Could you check a few things on this model? Use its own coordinates, in mm. A direction names the side the tool comes from. Round coordinates to 2 decimals unless told otherwise and drop trailing zeros. Loops run counter-clockwise (first coordinate to the right, second up) from the corner with the lowest first, then second, coordinate; pieces in that order, holes last. Notation, with made-up numbers: M 40.5,-9 L 61.5,-9 A34 ccw 61.5,30 Z; hole C 42,39 d9. An arc over 180 degrees is marked long. Return JSON: item names as keys, results as strings. Group by question number.
```python
from build123d import *

# Parameters (mm, degrees)
BODY_EXTRUDE_DEPTH         = 12
M4X0_7_TAPPED_HOLE6_D      = 3.3
CUT_EXTRUDE1_DEPTH         = 32.10064308
M3X0_5_TAPPED_HOLE1_REACH  = 33.101
M3X0_5_TAPPED_HOLE1_BORE_R = 1.25
CHAMFER1_SIZE              = 1


with BuildPart() as part:
    # Body Sketch → Body Extrude (new body)
    with BuildSketch(Plane.XY):
        Polygon((-26.5, 0), (26.5, 0), (26.5, 5), (4.5, 5), (4.5, 11), (-4.5, 11), (-4.5, 5), (-26.5, 5), align=None)
    extrude(amount=-BODY_EXTRUDE_DEPTH)

    # M4x0.7 Tapped Hole6 (through all)
    with Locations(Plane.XZ):
        with Locations((-22.5, -6), (22.5, -6)):
            Hole(M4X0_7_TAPPED_HOLE6_D / 2)

    # Sketch2 → Cut-Extrude1 (cut, through all)
    with BuildSketch(Plane(origin=(0, 0, 0), x_dir=(1, 0, 0), z_dir=(0, 1, 0))):
        with BuildLine():
            Line((-1.581929202, 4), (1.581929202, 4))
            ThreePointArc((1.581929202, 4), (0, 8.55), (-1.581929202, 4))
        make_face()
    extrude(amount=CUT_EXTRUDE1_DEPTH, mode=Mode.SUBTRACT)

    # M3x0.5 Tapped Hole1 bore → M3x0.5 Tapped Hole1 (cut, up to next)
    with BuildSketch(Plane.XY, mode=Mode.PRIVATE) as m3x0_5_tapped_hole1_sk1:
        with Locations((-22.5, 2.5)):
            Circle(M3X0_5_TAPPED_HOLE1_BORE_R)
    m3x0_5_tapped_hole1_tool1 = extrude(m3x0_5_tapped_hole1_sk1.sketch, amount=-M3X0_5_TAPPED_HOLE1_REACH, mode=Mode.PRIVATE) & part.part
    # M3x0.5 Tapped Hole1 bore → M3x0.5 Tapped Hole1 (cut, up to next)
    with BuildSketch(Plane.XY, mode=Mode.PRIVATE) as m3x0_5_tapped_hole1_sk2:
        with Locations((22.5, 2.5)):
            Circle(M3X0_5_TAPPED_HOLE1_BORE_R)
    m3x0_5_tapped_hole1_tool2 = extrude(m3x0_5_tapped_hole1_sk2.sketch, amount=-M3X0_5_TAPPED_HOLE1_REACH, mode=Mode.PRIVATE) & part.part
    # M3x0.5 Tapped Hole1 bore → M3x0.5 Tapped Hole1 (cut, up to next)
    with BuildSketch(Plane.XY, mode=Mode.PRIVATE) as m3x0_5_tapped_hole1_sk3:
        with Locations((0, 8)):
            Circle(M3X0_5_TAPPED_HOLE1_BORE_R)
    m3x0_5_tapped_hole1_tool3 = extrude(m3x0_5_tapped_hole1_sk3.sketch, amount=-M3X0_5_TAPPED_HOLE1_REACH, mode=Mode.PRIVATE) & part.part
    # M3x0.5 Tapped Hole1 bore → M3x0.5 Tapped Hole1 (cut, up to next)
    with BuildSketch(Plane.XY, mode=Mode.PRIVATE) as m3x0_5_tapped_hole1_sk4:
        with Locations((0, 3)):
            Circle(M3X0_5_TAPPED_HOLE1_BORE_R)
    m3x0_5_tapped_hole1_tool4 = extrude(m3x0_5_tapped_hole1_sk4.sketch, amount=-M3X0_5_TAPPED_HOLE1_REACH, mode=Mode.PRIVATE) & part.part
    add(m3x0_5_tapped_hole1_tool1.solids().sort_by_distance((-22.5, 2.5, 0))[0], mode=Mode.SUBTRACT)
    add(m3x0_5_tapped_hole1_tool2.solids().sort_by_distance((22.5, 2.5, 0))[0], mode=Mode.SUBTRACT)
    add(m3x0_5_tapped_hole1_tool3.solids().sort_by_distance((0, 8, 0))[0], mode=Mode.SUBTRACT)
    add(m3x0_5_tapped_hole1_tool4.solids().sort_by_distance((0, 3, 0))[0], mode=Mode.SUBTRACT)

    # Chamfer1
    chamfer1_edges = [part.edges().sort_by_distance(p)[0] for p in [
        (26.5, 2.5, 0),
        (-26.5, 2.5, 0),
        (26.5, 2.5, -12),
        (-26.5, 2.5, -12),
    ]]
    chamfer(chamfer1_edges, length=CHAMFER1_SIZE)


solid = part.part
```
1. If we section it at B-B, the plane x = 22.5: Please give me the cut outline in (y, z).
2. If we section it at A-A, the plane z = -6: Please give me the cut outline in (x, y).
3. I'm going to push flat-ended pins straight in: pin 1 Ø2 at (x, y) = (0, 8) entering from +Z; pin 2 Ø4 at (y, z) = (9.5, -5) entering from +X; pin 3 Ø3 at (y, z) = (7, -5.5) entering from -X. Where does each tip first touch, or does it pass through?
4. We'd pull the mould along Z, two halves only. Please class faces 5 (the face through (0, 11, -3)), 6 (the face through (-22.1, 2.5, -7.6)), 7 (the face through (26, 2.5, -0.5)): +Z half, -Z half, draft (parallel to the pull), parting line (faces both ways), or undercut.
5. I need wall thicknesses on probe 1 along X at (y, z) = (2.75, -3.5); probe 2 along X at (y, z) = (2, -7); probe 3 along Y at (x, z) = (-22.5, -3.5). Which ranges of each line are inside material? Lowest first, please.
6. If we section it at D-D, the plane y = 3: Please give me the cut outline in (x, z), then the cut area to 3 significant figures.
7. If we section it at C-C, the plane x = 0: Please give me the cut outline in (y, z), then the cut area to 4 significant figures.
8. On a 3-axis mill with a long thin cutter (end or side, diameter ignored), from which of +Z, -Z, +X, -X, +Y, -Y can I reach the whole of each face in a straight line? I mean faces 1 (the face through (-0.27, 6.78, -1.97)), 2 (the face through (-15, 5, -6)), 3 (the face through (16, 5, -6)), 4 (the face through (0, 5, -4)). Say none if no direction works.
Geometry results:
{
 "1": {"outline": "M 0,-12 L 5,-12 L 5,-7.65 L 0,-7.65 Z; M 0,-4.35 L 1.25,-4.35 L 1.25,0 L 0,0 Z; M 3.75,-4.35 L 5,-4.35 L 5,0 L 3.75,0 Z"},
 "2": {"outline": "M -26.5,0 L -24.15,0 L -24.15,5 L -26.5,5 Z; M -20.85,0 L -2.55,0 L -2.55,11 L -4.5,11 L -4.5,5 L -20.85,5 Z; M 2.55,0 L 20.85,0 L 20.85,5 L 4.5,5 L 4.5,11 L 2.55,11 Z; M 24.15,0 L 26.5,0 L 26.5,5 L 24.15,5 Z"},
 "3": {"pin 1": "z = -8.35", "pin 2": "x = 4.5", "pin 3": "x = -4.5"},
 "4": {"face 5": "draft", "face 6": "undercut", "face 7": "+Z half"},
 "5": {"probe 1": "-26.5 to -23.72, -21.28 to -1.22, 1.22 to 21.28, 23.72 to 26.5", "probe 2": "-26.5 to -23.81, -21.19 to -2.35, 2.35 to 21.19, 23.81 to 26.5", "probe 3": "0 to 1.25, 3.75 to 5"},
 "6": {"outline": "M -26.5,-11 L -25.5,-12 L 25.5,-12 L 26.5,-11 L 26.5,-1 L 25.5,0 L 23.65,0 L 23.65,-4.81 A1.65 cw long 21.35,-4.81 L 21.35,0 L 1.25,0 L 1.25,-4 L 1.58,-4 A2.55 cw long -1.58,-4 L -1.25,-4 L -1.25,0 L -21.35,0 L -21.35,-4.81 A1.65 cw long -23.65,-4.81 L -23.65,0 L -25.5,0 L -26.5,-1 Z", "area": "567 mm^2"},
 "7": {"outline": "M 0,-12 L 11,-12 L 11,-8.55 L 0,-8.55 Z; M 0,-4 L 1.75,-4 L 1.75,0 L 0,0 Z; M 4.25,-4 L 6.75,-4 L 6.75,0 L 4.25,0 Z; M 9.25,-4 L 11,-4 L 11,0 L 9.25,0 Z", "area": "61.95 mm^2"},
 "8": {"face 1": "+Z", "face 2": "+Z, -Z, -X, +Y", "face 3": "+Z, -Z, +X, +Y", "face 4": "+Y, -Y"}
}
